from build123d import *

# Parameters (mm, degrees)
SKICA1_R                 = 2
P_IDAT_VYSUNUT_M1_DEPTH  = 2
ODEBRAT_VYSUNUT_M1_DEPTH = 2
SKICA2_R                 = 1
P_IDAT_VYSUNUT_M2_DEPTH  = 6
ZKOSEN_1_SIZE            = 0.3
ZAOBLIT1_R               = 0.5


with BuildPart() as part:
    # Skica1 → Přidat vysunutím1 (new body)
    with BuildSketch(Plane.XY):
        Circle(SKICA1_R)
    extrude(amount=P_IDAT_VYSUNUT_M1_DEPTH)

    # Skica4 → Odebrat vysunutím1 (cut)
    with BuildSketch(Plane.XY.offset(2)):
        Polygon((-0.866025404, 0), (-0.433012702, -0.75), (0.433012702, -0.75), (0.866025404, 0), (0.433012702, 0.75), (-0.433012702, 0.75), align=None)
    extrude(amount=-ODEBRAT_VYSUNUT_M1_DEPTH, mode=Mode.SUBTRACT)

    # Skica2 → Přidat vysunutím2 (add)
    with BuildSketch(Plane(origin=(0, 0, 0), x_dir=(-1, 0, 0), z_dir=(0, 0, -1))):
        Circle(SKICA2_R)
    extrude(amount=P_IDAT_VYSUNUT_M2_DEPTH)

    # Zkosení1
    zkosen_1_edges = [part.edges().sort_by_distance(p)[0] for p in [
        (1, 0, -6),
    ]]
    chamfer(zkosen_1_edges, length=ZKOSEN_1_SIZE)

    # Zaoblit1
    zaoblit1_edges = [part.edges().sort_by_distance(p)[0] for p in [
        (-2, 0, 2),
    ]]
    fillet(zaoblit1_edges, radius=ZAOBLIT1_R)


solid = part.part
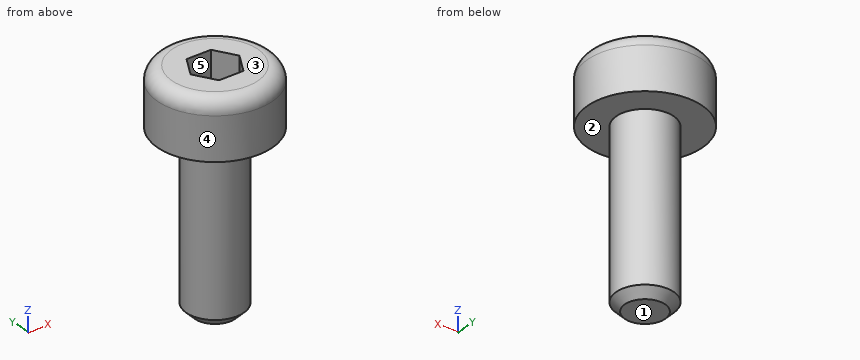
The listing builds one solid part. Answer for the finished solid, in the listing's coordinates (mm). Face numbers are marked on the shaded views. A direction names the side the tool comes from. Round coordinates to 2 decimals unless told otherwise and drop trailing zeros. Write each loop counter-clockwise with the first axis right and the second up, starting at its lowest first coordinate (ties: lowest second). Pieces come first, ordered by that corner, then holes. Notation, with made-up numbers: M 53.25,51 L 75.25,51 A34 ccw 75.25,90 Z; hole C 63,7.5 d10. An arc over 180 degrees is marked long. Write each question's results on one line, items separated by ' | '. Start each with the question number.
Item 1: Straight lines are drawn through the part: L1, parallel to Z at x = 0.75, y = 1; L2, parallel to Z at x = 0.4, y = 0.35; L3, parallel to X at y = 0.6, z = 1. For each, find the intervals that lie inside material, in ascending order. Write a range as [from, to].
Item 2: For the marked faces 1 and 2, determine the directions among +Z, -Z, +X, -X, +Y, -Y from which every point of the face is accessible in a straight line to the end or side of a thin tool.
Item 3: Flat-ended cylindrical pins translate along their axes: pin 1 Ø1 at (x, z) = (1, -1.5) entering from +Y; pin 2 Ø2 at (x, z) = (0, -5) entering from -Y; pin 3 Ø1 at (y, z) = (1, -5) entering from +X. Find the tip coordinate at first contact, or state that the pin passes through.
Item 4: A cutting plane is placed at A-A on x = 0. Write down the section's boundary in (y, z).
Item 5: A cutting plane is placed at B-B on z = -1.5. Write down the section's boundary in (x, y).
Item 6: For a pull along Y with two mould halves and no side action, classify the marked faces 3, 4 and 5 as pulls with the +Y half, pulls with the -Y half, needs draft (parallel to the pull), parting line crosses it, or undercut.
Check sheet entries:
1) L1: [0, 2] | L2: [-6, 0] | L3: [-1.91, -0.52], [0.52, 1.91]
2) face 1: -Z, +X, -X, +Y, -Y | face 2: -Z
3) pin 1: y = 0.87 | pin 2: y = -1 | pin 3: x = 0.87
4) outline: M -2,0 L -1,0 L -1,-5.7 L -0.7,-6 L 0.7,-6 L 1,-5.7 L 1,0 L 2,0 L 2,1.5 A0.5 ccw 1.5,2 L 0.75,2 L 0.75,0 L -0.75,0 L -0.75,2 L -1.5,2 A0.5 ccw -2,1.5 Z
5) outline: C 0,0 d2
6) face 3: needs draft | face 4: parting line crosses it | face 5: undercut
